The model under review builds one solid part; all positions refer to its coordinate system, in mm. A direction names the side the tool comes from. Coordinates: 2 decimals unless noted, no trailing zeros. Write each loop counter-clockwise with the first axis right and the second up, starting at its lowest first coordinate (ties: lowest second). Pieces come first, ordered by that corner, then holes. Notation, with made-up numbers: (-35, 44.5) - (-25, 44.5) arc R17 ccw to (-25, 50.5) - close; hole circle Ø3 at (81, -33). An arc over 180 degrees is marked (long way). Put each result on its own line as item: value. Start each with the question number.
Item 1: Consider section C-C on z = 3.5. Give the boundary of the cut face in (x, y), then the cut area to 4 significant figures.
Item 2: Consider section A-A on z = -18. Give the boundary of the cut face in (x, y).
Item 3: Machinability: for faces 1 (the face through (212, -10, -17)), 2 (the face through (212, -15, -22.4)), 3 (the face through (212, -5, 11.667)), which of the approach directions +Z, -Z, +X, -X, +Y, -Y give a long, thin tool a straight path to every point of the face, cutting with its end or side? Answer none if there is none.
Item 4: For pin 1 (1.5 mm diameter, centred on x = 279.5, z = -12, fed in from +Y); pin 2 (8 mm diameter, centred on x = 288, y = -14.5, fed in from +Z); pin 3 (8.5 mm diameter, centred on x = 240.5, z = -17, fed in from +Y), all flat-tipped, find the tip position at first contact; note any pin that passes through.
Item 5: Mouldability with a two-part tool opening along Y and no side actions: class faces 4 (the face through (120, 35, 0)), 5 (the face through (212, -5, -11.667)), 6 (the face through (222, 13, 31.267)) as pulls with the +Y half, pulls with the -Y half, needs draft (parallel to the pull), parting line crosses it, or undercut.
Item 6: Consider section B-B on x = 419. Give the boundary of the cut face in (y, z).
Item 7: To check wall thickness, follow L1, parallel to Y at x = 262, z = 8.5; L2, parallel to Y at x = 347, z = -24.5; L3, parallel to Y at x = 134, z = -27. State the ranges of each line that lie inside material, in increasing order. Write a range as [from, to].
```python
from build123d import *

# Parameters (mm, degrees)
BOSS_EXTRUDE1_DEPTH = 430
SKETCH1_3_W         = 62.533333334
SKETCH1_3_H         = 35
BOSS_EXTRUDE2_DEPTH = 450
CUT_EXTRUDE1_REACH  = 457.67


with BuildPart() as part:
    # Sketch1 → Boss-Extrude1 (new body)
    with BuildSketch(Plane(origin=(0, 0, 0), x_dir=(0, 0, -1), z_dir=(1, 0, 0))):
        Polygon((11.666666667, 0), (0, 0), (0, -20), (22.4, -20), (22.4, -10), (11.666666667, -10), align=None)
        Polygon((0, -20), (0, 0), (-11.666666667, 0), (-11.666666667, -10), (-22.4, -10), (-22.4, -20), align=None)
    extrude(amount=BOSS_EXTRUDE1_DEPTH)

    # Sketch1_3 → Boss-Extrude2 (add)
    with BuildSketch(Plane(origin=(0, 0, 0), x_dir=(0, 0, -1), z_dir=(1, 0, 0))):
        with Locations((0, 17.5)):
            Rectangle(SKETCH1_3_W, SKETCH1_3_H)
    extrude(amount=BOSS_EXTRUDE2_DEPTH)

    # Sketch2 → Cut-Extrude1 (cut, up to next)
    with BuildSketch(Plane.XY.offset(31.266666667), mode=Mode.PRIVATE) as cut_extrude1_sk1:
        Polygon((280.506060664, 35), (140.506060664, 35), (127, 20), (267, 20), align=None)
    cut_extrude1_tool1 = extrude(cut_extrude1_sk1.sketch, amount=-CUT_EXTRUDE1_REACH, mode=Mode.PRIVATE) & part.part
    # Sketch2 → Cut-Extrude1 (cut, up to next)
    with BuildSketch(Plane.XY.offset(31.266666667), mode=Mode.PRIVATE) as cut_extrude1_sk2:
        Polygon((0, 35), (0, 25), (100, 35), align=None)
    cut_extrude1_tool2 = extrude(cut_extrude1_sk2.sketch, amount=-CUT_EXTRUDE1_REACH, mode=Mode.PRIVATE) & part.part
    # Sketch2 → Cut-Extrude1 (cut, up to next)
    with BuildSketch(Plane.XY.offset(31.266666667), mode=Mode.PRIVATE) as cut_extrude1_sk3:
        Polygon((450, 35), (350, 35), (450, 25), align=None)
    cut_extrude1_tool3 = extrude(cut_extrude1_sk3.sketch, amount=-CUT_EXTRUDE1_REACH, mode=Mode.PRIVATE) & part.part
    add(cut_extrude1_tool1.solids().sort_by_distance((203.75303, 27.5, 31.266667))[0], mode=Mode.SUBTRACT)
    add(cut_extrude1_tool2.solids().sort_by_distance((33.333333, 31.666667, 31.266667))[0], mode=Mode.SUBTRACT)
    add(cut_extrude1_tool3.solids().sort_by_distance((416.666667, 31.666667, 31.266667))[0], mode=Mode.SUBTRACT)


solid = part.part
```
Report:
1. outline: (0, -20) - (430, -20) - (430, 0) - (450, 0) - (450, 25) - (350, 35) - (280.51, 35) - (267, 20) - (127, 20) - (140.51, 35) - (100, 35) - (0, 25) - close
1. area: 21,250 mm²
2. outline: (0, -20) - (430, -20) - (430, -10) - (0, -10) - close; (0, 0) - (450, 0) - (450, 25) - (350, 35) - (280.51, 35) - (267, 20) - (127, 20) - (140.51, 35) - (100, 35) - (0, 25) - close
3. face 1: -Z, +X, -X
3. face 2: -Z, +X, -X, -Y
3. face 3: +Z, +X, -X
4. pin 1: y = 34.72
4. pin 2: z = 22.4
4. pin 3: y = 20
5. face 4: pulls with the +Y half
5. face 5: undercut
5. face 6: needs draft
6. outline: (-20, -22.4) - (-10, -22.4) - (-10, -11.67) - (0, -11.67) - (0, -31.27) - (28.1, -31.27) - (28.1, 31.27) - (0, 31.27) - (0, 11.67) - (-10, 11.67) - (-10, 22.4) - (-20, 22.4) - close
7. L1: [-20, 20]
7. L2: [0, 35]
7. L3: [0, 20], [27.77, 35]
